The model under review builds one solid part; all positions refer to its coordinate system, in mm. Face numbers are marked on the shaded views. A direction names the side the tool comes from. Round coordinates to 2 decimals unless told otherwise and drop trailing zeros. Order: outer loops, then holes, each group sorted by start corner. A loop starts at its lowest first (then second) coordinate and runs counter-clockwise, first axis right, second up. Notation, with made-up numbers: (42.5, 13) - (51.5, 13) arc R29 cw to (51.5, 46) - close; hole circle Ø3 at (-32.5, 77). An arc over 180 degrees is marked (long way). One line per question, with ' | ' between items. Start each with the question number.
Item 1: Add section B-B on x = -28. State the section outline as (y, z) points.
Item 2: Tool access review of the marked faces 4, 5 and 6: name each direction out of +Z, -Z, +X, -X, +Y, -Y from which nothing blocks a thin tool from reaching the whole face with its end or side.
Item 3: For L1, parallel to X at y = 37, z = 10.25; L2, parallel to Z at x = 23, y = 30, list the stretches that pass through material, from the lowest coordinate up. Write a range as [from, to].
Item 4: Insertion check: pin 1 Ø2 at (x, y) = (-19.5, 16) entering from +Z; pin 2 Ø14 at (x, y) = (10, -14) entering from +Z; pin 3 Ø4 at (x, y) = (-20.5, -0.5) entering from -Z; pin 4 Ø5 at (y, z) = (43, 20.5) entering from +X. Each pin has a flat end and moves straight along its axis. Give the tip position at first contact, or say it passes through.
Item 5: Add section A-A on x = -9. State how many separate pieces and enclosed holes the cut face has, and give its area (3 significant figures).
Item 6: Draft analysis for pull direction Y (two halves, no side actions). For the marked faces 1, 2 and 3, state which applies: +Y half, -Y half, draft (parallel to the pull), parting line (faces both ways), or undercut.
from build123d import *

# Parameters (mm, degrees)
F1_DEPTH      = 31.75
F2_W          = 52.7695193887
F2_H          = 120.6567846239
F3_DEPTH      = 25.4
F4_W          = 44.4975402206
F4_H          = 18.5406431556
F5_DEPTH      = 25.4
F6_W          = 34.7439497709
F6_H          = 5.4911417693
F7_DEPTH      = 54.31181
F8_W          = 12.1364339493
F8_H          = 2.9900523731
F9_DEPTH      = 56.69838
F10_W         = 22.7860264232
F10_H         = 8.4337261604
F11_DEPTH     = 56.06512
F12_T1_DEPTH  = 52.7695193887
F12_T6_DEPTH  = 52.7695193887
F12_T11_DEPTH = 52.7695193887
F14_DEPTH     = 55.98348
F15_T1_DEPTH  = 52.7695193887
F16_R         = 7.2468545108
F17_DEPTH     = 4.48168
F19_SIZE      = 5.08
F20_T1_DEPTH  = 149.6281885647
F21_R         = 6.1019617507
F22_DEPTH     = 3.60881
F24_R         = 2.6289
F25_DEPTH     = 82.93478
F26_DEPTH     = 96.11065
F27_W         = 7.3527656496
F27_H         = 7.1394555271
F28_DEPTH     = 1.80312
F29_DEPTH     = 3.46127
F30_W         = 7.1394555271
F30_H         = 2.632195
F31_DEPTH     = 6.31406


# Not quite as in the source:
# - a fillet or chamfer that OpenCascade refuses, or shapes differently, is made with other operations: its cross-section is extruded or revolved along the edge and cut away or added


with BuildPart() as f1:
    # F0 (on Right) → F1 (new body, symmetric)
    with BuildSketch(Plane.YZ):
        Polygon((55.6219257414, 26.0995179415), (-71.0249170661, 0), (55.6219257414, 0), align=None)
    extrude(amount=F1_DEPTH, both=True)

    # F2 (on face) → F3 (cut)
    with BuildSketch(Plane(origin=(0, 0, 0), x_dir=(1, 0, 0), z_dir=(0, 0, -1))):
        with Locations((0.7131025195, 7.7014956623)):
            Rectangle(F2_W, F2_H)
    extrude(amount=-F3_DEPTH, mode=Mode.SUBTRACT)

    # F4 (on face) → F5 (cut)
    with BuildSketch(Plane.XZ.offset(-52.6268966496)):
        with Locations((0.5704807118, 11.6948671639)):
            Rectangle(F4_W, F4_H)
    extrude(amount=-F5_DEPTH, mode=Mode.SUBTRACT)

    # F6 (on face) → F7 (join)
    with BuildSketch(Plane.YZ.offset(-25.6716571748)):
        with Locations((17.3719748855, 11.8913206175)):
            Rectangle(F6_W, F6_H)
    extrude(amount=F7_DEPTH)

    # F8 (on face) → F9 (join)
    with BuildSketch(Plane.YZ.offset(-25.6716571748)):
        with Locations((-6.0682169747, 10.6407759194)):
            Rectangle(F8_W, F8_H)
    extrude(amount=F9_DEPTH)

    # F10 (on face) → F11 (join)
    with BuildSketch(Plane.YZ.offset(-25.6716571748)):
        with Locations((-18.7075927729, 4.2168630802)):
            Rectangle(F10_W, F10_H)
    extrude(amount=F11_DEPTH)

    # F12: chamfer of 5.08 on 3 edges, made by hand

    # F12_s2 → F12_t1 (cut)
    with BuildSketch(Plane.YZ.offset(-25.6716571748)):
        Polygon((-30.1006059845, 3.3537261604), (-25.0206059845, 8.4337261604), (-30.1006059845, 8.4337261604), align=None)
    extrude(amount=F12_T1_DEPTH, mode=Mode.SUBTRACT)


with BuildPart() as f12_tool4:
    # F12_s5 → F12_t6 (new body)
    with BuildSketch(Plane.YZ.offset(-25.6716571748)):
        Polygon((5.08, 14.6368915021), (0, 9.5568915021), (0, 14.6368915021), align=None)
    extrude(amount=F12_T6_DEPTH)

    split(bisect_by=Plane.XY.offset(12.1358021059), keep=Keep.TOP)


with BuildPart() as f1_1:
    add(f1.part)

    # F12_t3: cut F12_tool4
    add(f12_tool4.part, mode=Mode.SUBTRACT)


with BuildPart() as f12_tool9:
    # F12_s10 → F12_t11 (new body)
    with BuildSketch(Plane.YZ.offset(-25.6716571748)):
        Polygon((-12.1364339493, 7.0558021059), (-7.0564339493, 12.1358021059), (-12.1364339493, 12.1358021059), align=None)
    extrude(amount=F12_T11_DEPTH)

    split(bisect_by=Plane.XY.offset(8.4337261604), keep=Keep.TOP)


with BuildPart() as f1_2:
    add(f1_1.part)

    # F12_t8: cut F12_tool9
    add(f12_tool9.part, mode=Mode.SUBTRACT)

    # F13 (on face) → F14 (join)
    with BuildSketch(Plane.YZ.offset(-25.6716571748)):
        Polygon((-68.0298879743, 0), (-44.0034680068, 0), (-44.0034680068, 3.4875369165), (-54.1017868902, 3.4875369165), (-68.0298879743, 0.6172188251), align=None)
    extrude(amount=F14_DEPTH)

    # F15: chamfer of 5.08 on 1 edges, made by hand

    # F15_s2 → F15_t1 (cut)
    with BuildSketch(Plane.YZ.offset(-25.6716571748)):
        with BuildLine():
            Line((-59.2793850519, 2.4415783127), (-48.81963513, 3.5081501604))
            Line((-48.81963513, 3.5081501604), (-48.81963513, 3.6097501604))
            ThreePointArc((-48.81963513, 3.6097501604), (-51.4607110101, 3.5891369165), (-54.1017868902, 3.5891369165))
            Line((-54.1017868902, 3.5891369165), (-54.1222937974, 3.5870458445))
            ThreePointArc((-54.1222937974, 3.5870458445), (-56.7090125934, 3.0539720456), (-59.2998919591, 2.5410872407))
            Line((-59.2998919591, 2.5410872407), (-59.2793850519, 2.4415783127))
        make_face()
    extrude(amount=F15_T1_DEPTH, mode=Mode.SUBTRACT)

    # F16 (on face) → F17 (join)
    with BuildSketch(Plane.XY.offset(14.6368915021)):
        with Locations((15.2392005548, 17.7897959948)):
            Circle(F16_R)
    extrude(amount=F17_DEPTH)

    # F18: fillet of radius 5.08 on 1 edges, made by hand

    # F18_s1 → F18_t2 (revolve, cut)
    with BuildSketch(Plane.XZ.offset(-17.7897959948)):
        with BuildLine():
            ThreePointArc((22.4860550656, 14.6368915021), (20.8153524575, 17.8363251539), (17.4414130389, 19.1185715021))
            Line((17.4414130389, 19.1185715021), (22.4860550656, 19.1185715021))
            Line((22.4860550656, 19.1185715021), (22.4860550656, 14.6368915021))
        make_face()
    revolve(axis=Axis((15.2392005548, 17.7897959948, 19.1185715021), (0, 0, 1)), mode=Mode.SUBTRACT)

    # F19
    f19_edges = [f1_2.edges().sort_by_distance(p)[0] for p in [
        (0, -71.024917, 0),
    ]]
    chamfer(f19_edges, length=F19_SIZE)

    # F20: fillet of radius 5.08 on 2 edges, made by hand

    # F20_s2 → F20_t1 (cut)
    with BuildSketch(Plane(origin=(0, 70.954042843, 14.6222856658), x_dir=(1, 0, 0), z_dir=(0, -0.9794185829, -0.2018396378))):
        with BuildLine():
            ThreePointArc((-26.67, 14.3356435337), (-30.2621024484, 12.8477459822), (-31.75, 9.2556435337))
            Line((-31.75, 9.2556435337), (-31.75, 14.3356435337))
            Line((-31.75, 14.3356435337), (-26.67, 14.3356435337))
        make_face()
        with BuildLine():
            ThreePointArc((26.67, 14.3356435337), (30.2621024484, 12.8477459822), (31.75, 9.2556435337))
            Line((31.75, 9.2556435337), (31.75, 14.3356435337))
            Line((31.75, 14.3356435337), (26.67, 14.3356435337))
        make_face()
    extrude(amount=F20_T1_DEPTH, mode=Mode.SUBTRACT)

    # F21 (on face) → F22 (join)
    with BuildSketch(Plane.XY.offset(14.6368915021)):
        with Locations((-19.1379822791, 16.5131352842)):
            Circle(F21_R)
    extrude(amount=F22_DEPTH)

    # F23: fillet of radius 5.08 on 1 edges, made by hand

    # F23_s1 → F23_t2 (revolve, cut)
    with BuildSketch(Plane.XZ.offset(-16.5131352842)):
        with BuildLine():
            ThreePointArc((-13.0360205283, 14.6368915021), (-14.8707219244, 17.2449198831), (-17.8983245073, 18.2457015021))
            Line((-17.8983245073, 18.2457015021), (-13.0360205283, 18.2457015021))
            Line((-13.0360205283, 18.2457015021), (-13.0360205283, 14.6368915021))
        make_face()
    revolve(axis=Axis((-19.1379822791, 16.5131352842, 18.2457015021), (0, 0, 1)), mode=Mode.SUBTRACT)

    # F24 (on face) → F25 (cut)
    with BuildSketch(Plane.YZ.offset(31.75)):
        with Locations((-7.8780742586, 3.2512)):
            Circle(F24_R)
    extrude(amount=-F25_DEPTH, mode=Mode.SUBTRACT)

    # F24 (on face) → F26 (cut, symmetric)
    with BuildSketch(Plane.YZ.offset(31.75)):
        with Locations((-7.8780742586, 3.2512)):
            Circle(F24_R)
        with Locations((42.9219257414, 3.2512)):
            Circle(F24_R)
    extrude(amount=F26_DEPTH, both=True, mode=Mode.SUBTRACT)

    # F27 (on face) → F28 (join)
    with BuildSketch(Plane.XY.offset(14.6368915021)):
        with Locations((-2.9632803053, 31.1742220074)):
            Rectangle(F27_W, F27_H)
    extrude(amount=F28_DEPTH)

    # F29 (add): a face of the model
    f29_faces = [f1_2.faces().sort_by_distance(p)[0] for p in [
        (-2.9632803053, 31.1742220074, 16.4400115021),
    ]]
    extrude(f29_faces, amount=F29_DEPTH)

    # F30 (on face) → F31 (join)
    with BuildSketch(Plane.YZ.offset(0.7131025195)):
        with Locations((31.1742220074, 18.5851840021)):
            Rectangle(F30_W, F30_H)
    extrude(amount=F31_DEPTH)


solid = f1_2.part
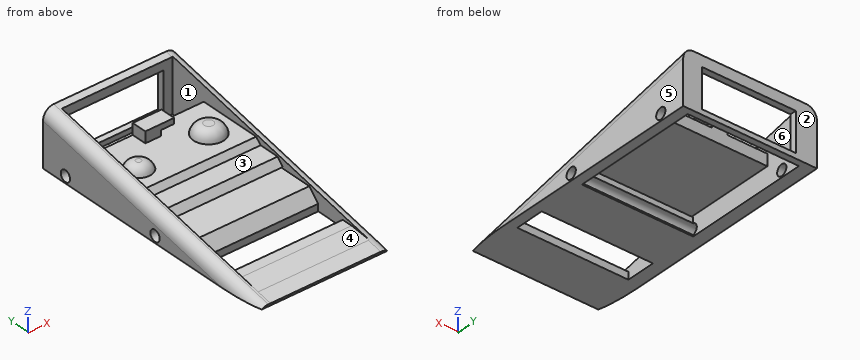
Determined:
1) outline: (-66.03, 0.85) - (-65.94, 0) - (55.62, 0) - (55.62, 25.92) - close; hole circle Ø5.26 at (-7.88, 3.25); hole circle Ø5.26 at (42.92, 3.25)
2) face 4: +Z, -Y | face 5: +Z, -Z, +X, +Y, -Y | face 6: none
3) L1: [-31.75, -25.67], [27.1, 31.75] | L2: [9.15, 14.64]
4) pin 1: z = 18.25 | pin 2: z = 12.14 | pin 3: z = 9.15 | pin 4: x = 31.75
5) separate pieces: 5 | enclosed holes: 0 | area: 453 mm2
6) face 1: undercut | face 2: +Y half | face 3: draft
